```python
from build123d import *

# Parameters (mm, degrees)
BOSS_EXTRUDE1_DEPTH      = 6
SKETCH3_R                = 6
BOSS_EXTRUDE2_DEPTH      = 14
BOSS_EXTRUDE3_DEPTH      = 6
BOSS_EXTRUDE3_DEPTH_BACK = 6
SKETCH5_R                = 5
CUT_EXTRUDE1_DEPTH       = 13.536489687
SKETCH6_R                = 4.9
CUT_EXTRUDE2_DEPTH       = 20


with BuildPart() as part:
    # Sketch2 → Boss-Extrude1 (new body)
    with BuildSketch(Plane(origin=(0, 0, 0), x_dir=(1, 0, 0), z_dir=(0, 1, 0))):
        with BuildLine():
            Line((-3.80541246, 6.462881402), (3.677540288, 6.536489687))
            ThreePointArc((3.677540288, 6.536489687), (7.499909291, 0.03688665), (3.741657387, -6.5))
            Line((3.741657387, -6.5), (-3.741657387, -6.5))
            ThreePointArc((-3.741657387, -6.5), (-7.499909291, -0.03688665), (-3.80541246, 6.462881402))
        make_face()
    extrude(amount=BOSS_EXTRUDE1_DEPTH)

    # Sketch3 → Boss-Extrude2 (add)
    with BuildSketch(Plane(origin=(0, 6, 0), x_dir=(1, 0, 0), z_dir=(0, 1, 0))):
        Circle(SKETCH3_R)
    extrude(amount=BOSS_EXTRUDE2_DEPTH)

    # Sketch4 → Boss-Extrude3 (add, two sides)
    with BuildSketch(Plane.XY) as boss_extrude3_sk:
        with BuildLine():
            Line((6, 20), (9.551839137, 24.736029469))
            ThreePointArc((9.551839137, 24.736029469), (0.00015174, 44), (-9.551535656, 24.736029469))
            Line((-9.551535656, 24.736029469), (-6, 20))
            Line((-6, 20), (-4.800072834, 18.400029674))
            ThreePointArc((-4.800072834, 18.400029674), (0, 15.999932561), (4.800072834, 18.400029674))
            Line((4.800072834, 18.400029674), (6, 20))
        make_face()
    extrude(amount=BOSS_EXTRUDE3_DEPTH)
    extrude(boss_extrude3_sk.sketch, amount=-BOSS_EXTRUDE3_DEPTH_BACK)

    # Sketch5 → Cut-Extrude1 (cut, through all)
    with BuildSketch(Plane.XY.offset(6)):
        with Locations((0.00015174, 32)):
            Circle(SKETCH5_R)
    extrude(amount=-CUT_EXTRUDE1_DEPTH, mode=Mode.SUBTRACT)

    # Sketch6 → Cut-Extrude2 (cut)
    with BuildSketch(Plane.XZ):
        Circle(SKETCH6_R)
    extrude(amount=-CUT_EXTRUDE2_DEPTH, mode=Mode.SUBTRACT)


solid = part.part
```
For this review, take the finished solid that the model builds, in its own axes (mm). A direction names the side the tool comes from. Coordinates: 2 decimals unless noted, no trailing zeros. Write each loop counter-clockwise with the first axis right and the second up, starting at its lowest first coordinate (ties: lowest second). Pieces come first, ordered by that corner, then holes. Notation, with made-up numbers: (45, 28) - (86, 28) arc R9 cw to (86, 45) - close; hole circle Ø6 at (48, 14.5). An arc over 180 degrees is marked (long way). Answer in a Markdown table with one row per item. Add a question column.
Q1. Tool access review of faces 1 (the flat face through (2, 27, -6)), 2 (the cylindrical face through (-3.894, 17.435, 5.239)), 3 (the cylindrical face through (-3.894, 17.435, -5.239)): name each direction out of +Z, -Z, +X, -X, +Y, -Y from which nothing blocks a thin tool from reaching the whole face with its end or side.
Q2. For P1, Ø1.5, axis at y = 29.5, z = -2, coming from the +X side; P2, Ø4, axis at y = 37.5, z = -1.5, coming from the -X side; P3, Ø1, axis at x = -2, z = 0, coming from the +Y side; P4, Ø7, axis at x = -1, y = 32, coming from the +Z side, all flat-tipped, find the tip position at first contact; note any pin that passes through.
Q3. We need section C-C, the plane z = 2.75. State the section outline as (x, y) points.
Q4. For probe 1 along Z at (x, y) = (-0.25, 15); probe 2 along Y at (x, z) = (0, -2.5); probe 3 along Z at (x, y) = (0.75, 37), list the stretches that pass through material, from the lowest coordinate up.
Q5. We need section B-B, the plane x = -1. State the section outline as (y, z) points.
Q6. Draft analysis for pull direction X (two halves, no side actions). For faces 4 (the cylindrical face through (0, 44, 0)), 5 (the cylindrical face through (-1.062, 9.86, -4.783)), 6 (the flat face through (0, 20, 0)), 7 (the cylindrical face through (3.874, 17.418, -5.15)), state which applies: +X half, -X half, draft (parallel to the pull), parting line (faces both ways), or undercut.
Q7. We need section A-A, the plane y = 32. State the section outline as (x, z) points, and give its area (3 significant figures).
Q8. We need section D-D, the plane x = 2. State the section outline as (y, z) points, and give its area (3 significant figures).
Answer list:
| question | item | result |
|---|---|---|
| 1 | face 1 | -Z, +X, -X, +Y |
| 1 | face 2 | +Z, -X |
| 1 | face 3 | -Z, -X |
| 2 | P1 | stops at x = 11.87 |
| 2 | P2 | stops at x = -11.48 |
| 2 | P3 | stops at y = 43.91 |
| 2 | P4 | passes through |
| 3 | outline | (-9.55, 24.74) - (-6, 20) - (-5.33, 19.11) - (-5.33, 6) - (-6.98, 6) - (-6.98, 0) - (-4.06, 0) - (-4.06, 20) - (4.06, 20) - (4.06, 0) - (6.98, 0) - (6.98, 6) - (5.33, 6) - (5.33, 19.11) - (6, 20) - (9.55, 24.74) arc R12 ccw (long way) to start; hole circle Ø10 at (0, 32) |
| 4 | probe 1 | z = -5.99 to -4.89, 4.89 to 5.99 |
| 4 | probe 2 | y = 20 to 27, 37 to 44 |
| 4 | probe 3 | z = -6 to 6 |
| 5 | outline | (0, -6.49) - (6, -6.49) - (6, -5.92) - (16.08, -5.92) - (16.08, -6) - (27.1, -6) - (27.1, 6) - (16.08, 6) - (16.08, 5.92) - (6, 5.92) - (6, 6.5) - (0, 6.5) - (0, 4.8) - (20, 4.8) - (20, -4.8) - (0, -4.8) - close; (36.9, -6) - (43.96, -6) - (43.96, 6) - (36.9, 6) - close |
| 6 | face 4 | parting line |
| 6 | face 5 | undercut |
| 6 | face 6 | undercut |
| 6 | face 7 | +X half |
| 7 | outline | (-12, -6) - (-5, -6) - (-5, 6) - (-12, 6) - close; (5, -6) - (12, -6) - (12, 6) - (5, 6) - close |
| 7 | area | 168 mm2 |
| 8 | outline | (0, -6.52) - (6, -6.52) - (6, -5.66) - (16.34, -5.66) - (16.34, -6) - (27.42, -6) - (27.42, 6) - (16.34, 6) - (16.34, 5.66) - (6, 5.66) - (6, 6.5) - (0, 6.5) - (0, 4.47) - (20, 4.47) - (20, -4.47) - (0, -4.47) - close; (36.58, -6) - (43.83, -6) - (43.83, 6) - (36.58, 6) - close |
| 8 | area | 236 mm2 |
